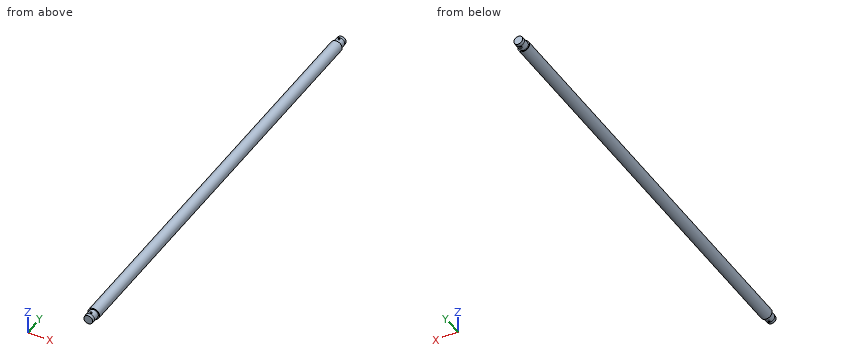
Solid Edge part; units mm, degrees
sketch "Sketch1" plane through (0, 0, 0) normal (1, 0, 0) x (0, 1, 0)
  line L0 (-234, 0) -> (-234, 4.5)
  line L1 (-234, 4.5) -> (-231, 4.8)
  line L2 (-231, 4.8) -> (-224, 4.8)
  line L3 (-224, 4.8) -> (-224, 6)
  line L4 (-224, 6) -> (0, 6)
  line L5 (0, 6) -> (0, 0)
  dimension "D1" = 234
revolve "RevolvedProtrusion1" add sketch "Sketch1" angle 360 about axis through (0, -238, 0) along (0, 1, 0)
mirror "Mirror1" about plane through (0, 0, 0) normal (0, -1, 0) of "RevolvedProtrusion1"
hole "Hole1" at (0, -229, 0) direction (0, 0, 1) diameter 2.254 end through all
hole "Hole2" at (0, 229, 0) direction (0, 0, 1) diameter 2.254 end through all
mirror "Mirror2" about plane through (0, 0, 0) normal (0, 0, 1) of "Hole1", "Hole2"
properties part number "19" material "Aluminiumlegierung:3.0205, Al 99.0, EN-AW 1200"
Could you check a few things on this model? Use its own coordinates, in mm. Coordinates: 2 decimals unless noted, no trailing zeros. Loops run counter-clockwise (first coordinate to the right, second up) from the corner with the lowest first, then second, coordinate; pieces in that order, holes last. Notation, with made-up numbers: M 79.25,-22 L 122.25,-22 A21 ccw 122.25,-9 Z; hole C 89,78 d8. An arc over 180 degrees is marked long. Put each result on its own line as item: value. Start each with the question number.
(1) I need wall thicknesses on line 1 (Y direction, x = 0, z = 3.75); line 2 (X direction, y = 229, z = 1.75); line 3 (X direction, y = -229, z = 2.25). Which ranges of each line are inside material? Lowest first, please. Write a range as from..to.
(2) Suppose I cut it at A-A on y = -26. Please give me the cut outline in (x, z).
(3) Will these pins go through, and if not, where does the flat tip stop? P1, Ø3, axis at x = 0, y = -229, coming from the +Z side; P2, Ø1.5, axis at y = 10, z = -2.5, coming from the +X side; P3, Ø2, axis at y = -89, z = -4, coming from the -X side.
(4) Suppose I cut it at B-B on z = -0.75. Count the separate pieces of the cut face and the enclosed holes in it, then the cut area to 3 significant figures.
Solutions:
1. line 1: y = -234..-230.13, -227.87..227.87, 230.13..234
1. line 2: x = -4.47..-1.13, 1.13..4.47
1. line 3: x = -4.24..-1.13, 1.13..4.24
2. outline: C 0,0 d12
3. P1: stops at z = 4.8
3. P2: stops at x = 5.74
3. P3: stops at x = -5.2
4. separate pieces: 1
4. enclosed holes: 2
4. area: 5,510 mm2
